Design review of the part built by this model. Coordinates are the model's own, in mm. Face numbers are marked on the shaded views. A direction names the side the tool comes from. Give positions to 0.01 mm unless a question says otherwise; leave off trailing zeros. Write each loop counter-clockwise with the first axis right and the second up, starting at its lowest first coordinate (ties: lowest second). Pieces come first, ordered by that corner, then holes. Notation, with made-up numbers: (-12.5, 31) -> (36.5, 31) arc R22 ccw to (36.5, 44) -> close; hole circle Ø3 at (-7, 69). An arc over 180 degrees is marked (long way). Write each question's results on one line, items separated by ' | '. Start each with the question number.
(1) Take a section at C-C (z = 8). State the section outline as (x, y) points, plus the area to 3 significant figures.
(2) Mouldability with a two-part tool opening along X and no side actions: class the marked faces 1, 2, 3 and 4 as released by +X, released by -X, zero draft, split by the parting line, or undercut.
(3) Clearance check with flat-ended pins moving along their axes: pin 1 (3 mm diameter, centred on y = -0.5, z = 9, fed in from -X); pin 2 (1.8 mm diameter, centred on x = -1, y = 0.5, fed in from +Z); pin 3 (1.8 mm diameter, centred on y = -1, z = 10.5, fed in from +X). State where each tip first meets the part, or that it passes through.
(4) To check wall thickness, follow probe 1 along X at (y, z) = (0.7, 7.25); probe 2 along X at (y, z) = (1.2, 1.5); probe 3 along Z at (x, y) = (9, 2.65). State the ranges of each line that lie inside material, in increasing order.
(5) For the marked faces 5, 6, 7, 8 and 9, list the 3-axis set-ups (+Z, -Z, +X, -X, +Y, -Y) from which the entire face can be reached by the end or side of a thin tool; tool diameter is ignored.
(6) Take a section at A-A (z = 2). State the section outline as (x, y) points.
(7) Take a section at B-B (y = 0.95). State the section outline as (x, z) points, plus the area to 3 significant figures.
(8) Take a section at D-D (x = -10). State the section outline as (y, z) points, plus the area to 3 significant figures.
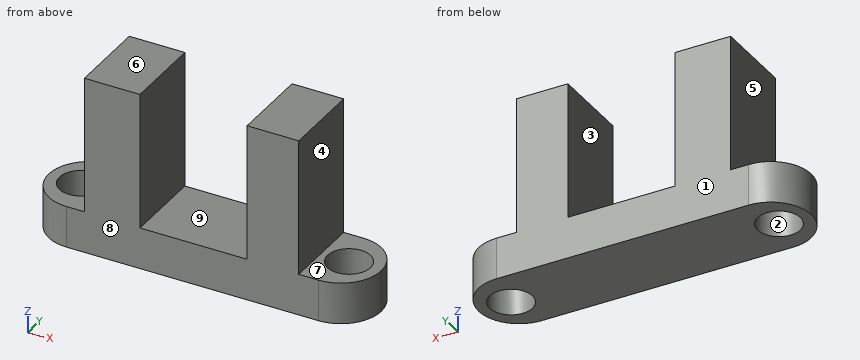
from build123d import *

# Parameters (mm, degrees)
F0_R     = 1.6
F1_DEPTH = 3.1
F3_DEPTH = 10.2


with BuildPart() as f1:
    # F0 (on Top) → F1 (new body)
    with BuildSketch(Plane.XY):
        with BuildLine():
            ThreePointArc((12.4, 0), (11.5213203436, 2.1213203436), (9.4, 3))
            Line((9.4, 3), (-9.4, 3))
            ThreePointArc((-9.4, 3), (-11.5213203436, 2.1213203436), (-12.4, 0))
            ThreePointArc((-12.4, 0), (-11.5213203436, -2.1213203436), (-9.4, -3))
            Line((-9.4, -3), (9.4, -3))
            ThreePointArc((9.4, -3), (11.5213203436, -2.1213203436), (12.4, 0))
        make_face()
        with Locations((-10, 0)):
            Circle(F0_R, mode=Mode.SUBTRACT)
        with BuildLine():
            ThreePointArc((11.6, 0), (10, -1.6), (8.4, 0))
            ThreePointArc((8.4, 0), (10, 1.6), (11.6, 0))
        make_face(mode=Mode.SUBTRACT)
    extrude(amount=F1_DEPTH)

    # F2 (on face) → F3 (join)
    with BuildSketch(Plane.XY.offset(3.1)):
        Polygon((-3.9267988071, -3), (-3.9267988071, 0), (-3.9267988071, 3), (-8.0732011929, 3), (-8.0732011929, -3), align=None)
        Polygon((4.0732011929, 3), (4.0732011929, 0), (4.0732011929, -3), (7.9267988071, -3), (7.9267988071, 3), align=None)
    extrude(amount=F3_DEPTH)


solid = f1.part
Report:
1) outline: (-8.07, -3) -> (-3.93, -3) -> (-3.93, 3) -> (-8.07, 3) -> close; (4.07, -3) -> (7.93, -3) -> (7.93, 3) -> (4.07, 3) -> close | area: 48.0 mm2
2) face 1: zero draft | face 2: undercut | face 3: undercut | face 4: released by +X
3) pin 1: x = -8.07 | pin 2: z = 3.1 | pin 3: x = 7.93
4) probe 1: -8.07 to -3.93, 4.07 to 7.93 | probe 2: -12.15 to -11.06, -8.94 to 8.94, 11.06 to 12.15 | probe 3: 0 to 3.1
5) face 5: +Z, -X, +Y, -Y | face 6: +Z, +X, -X, +Y, -Y | face 7: +Z, +X, +Y, -Y | face 8: +Z, -Z, +X, -X, -Y | face 9: +Z, +Y, -Y
6) outline: (-9.4, -3) -> (9.4, -3) arc R3 ccw to (9.4, 3) -> (-9.4, 3) arc R3 ccw to start; hole circle Ø3.2 at (-10, 0); hole circle Ø3.2 at (10, 0)
7) outline: (-12.25, 0) -> (-11.29, 0) -> (-11.29, 3.1) -> (-12.25, 3.1) -> close; (-8.71, 0) -> (8.71, 0) -> (8.71, 3.1) -> (7.93, 3.1) -> (7.93, 13.3) -> (4.07, 13.3) -> (4.07, 3.1) -> (-3.93, 3.1) -> (-3.93, 13.3) -> (-8.07, 13.3) -> (-8.07, 3.1) -> (-8.71, 3.1) -> close; (11.29, 0) -> (12.25, 0) -> (12.25, 3.1) -> (11.29, 3.1) -> close | area: 142 mm2
8) outline: (-2.94, 0) -> (-1.6, 0) -> (-1.6, 3.1) -> (-2.94, 3.1) -> close; (1.6, 0) -> (2.94, 0) -> (2.94, 3.1) -> (1.6, 3.1) -> close | area: 8.30 mm2
